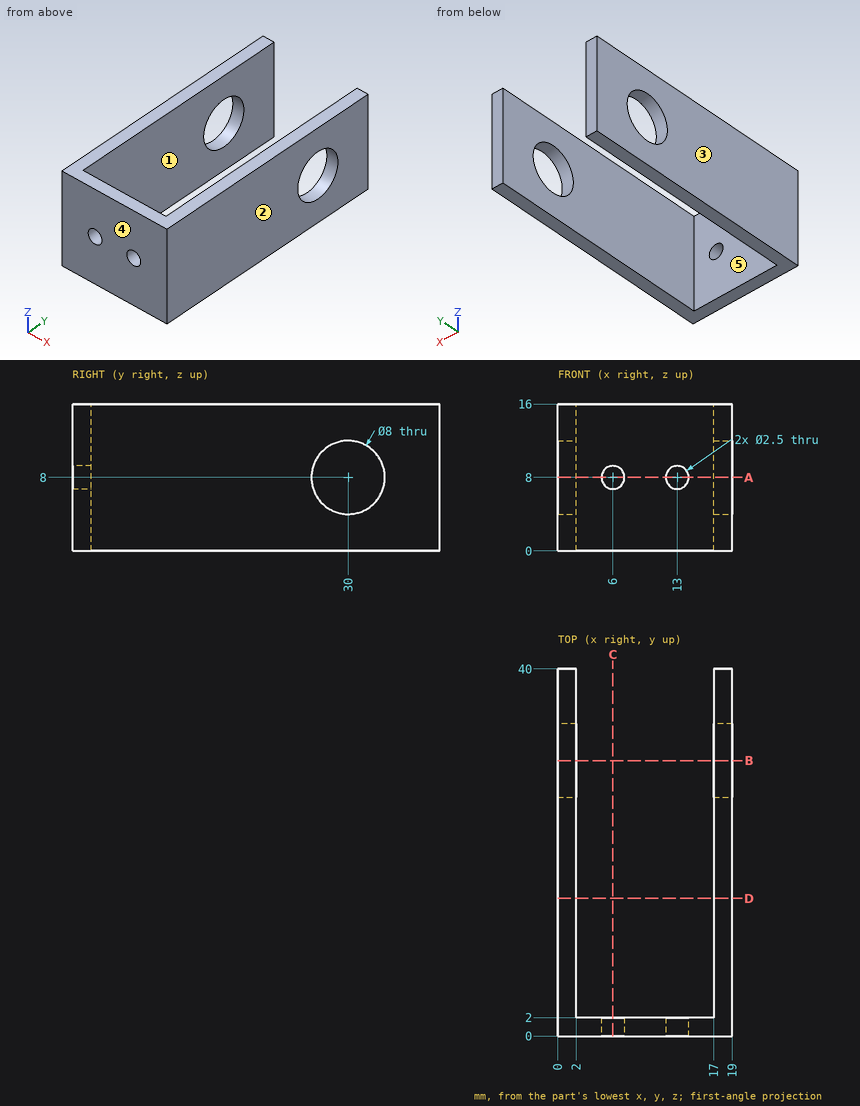
The figure shows three views and two pictorial views of one solid part (mm, origin at its lowest corner). Answer the questions. A direction names the side the tool comes from. Give positions to 0.01 mm unless a question says otherwise; leave off trailing zeros. Order: outer loops, then holes, each group sorted by start corner. A loop starts at its lowest first (then second) coordinate and runs counter-clockwise, first axis right, second up. Notation, with made-up numbers: M -26,81 L 7,81 A28 cw 7,115 Z; hole C 61.25,32.5 d8. An arc over 180 degrees is marked long. Return JSON: item names as keys, results as strings.
1) Section D-D, the plane y = 15 is taken. Write down the section's boundary in (x, z), plus the area to 3 significant figures.
Resolved:
{"outline": "M 0,0 L 2,0 L 2,16 L 0,16 Z; M 17,0 L 19,0 L 19,16 L 17,16 Z", "area": "64.0 mm^2"}
2) Section C-C, the plane x = 6 is taken. Write down the section's boundary in (y, z).
Resolved:
{"outline": "M 0,0 L 2,0 L 2,6.75 L 0,6.75 Z; M 0,9.25 L 2,9.25 L 2,16 L 0,16 Z"}
3) For a pull along X with two mould halves and no side action, classify the marked faces 3, 4 and 5 as +X half, -X half, draft (parallel to the pull), parting line (faces both ways), or undercut.
Resolved:
{"face 3": "-X half", "face 4": "draft", "face 5": "undercut"}
4) Section A-A, the plane z = 8 is taken. Write down the section's boundary in (x, y), plus the area to 3 significant figures.
Resolved:
{"outline": "M 0,0 L 4.75,0 L 4.75,2 L 2,2 L 2,26 L 0,26 Z; M 0,34 L 2,34 L 2,40 L 0,40 Z; M 7.25,0 L 11.75,0 L 11.75,2 L 7.25,2 Z; M 14.25,0 L 19,0 L 19,26 L 17,26 L 17,2 L 14.25,2 Z; M 17,34 L 19,34 L 19,40 L 17,40 Z", "area": "148 mm^2"}
5) Straight lines are drawn through the part: line 1 along Z through (x, y) = (17.65, 30); line 2 along X through (y, z) = (8, 8.25); line 3 along Y through (x, z) = (7, 10.5). For each, find the intervals that lie inside material, in ascending order. Write a range as [from, to].
Resolved:
{"line 1": "[0, 4], [12, 16]", "line 2": "[0, 2], [17, 19]", "line 3": "[0, 2]"}
6) A tool of negligible diameter and unlimited length cuts with its end or side. For the marked faces 1 and 2, from which of +Z, -Z, +X, -X, +Y, -Y can it reach the whole face along a straight path? Write none if from no direction.
Resolved:
{"face 1": "+Z, -Z, +Y", "face 2": "+Z, -Z, +X, +Y, -Y"}
7) Each of these flat-tipped pins is pushed along its axis until it touches: pin 1 (4 mm diameter, centred on x = 13, z = 7, fed in from +Y); pin 2 (4 mm diameter, centred on y = 29, z = 8, fed in from -X). Where does it stop, or does it pass through?
Resolved:
{"pin 1": "y = 2", "pin 2": "through"}
8) Section B-B, the plane y = 30 is taken. Write down the section's boundary in (x, z), plus the area to 3 significant figures.
Resolved:
{"outline": "M 0,0 L 2,0 L 2,4 L 0,4 Z; M 0,12 L 2,12 L 2,16 L 0,16 Z; M 17,0 L 19,0 L 19,4 L 17,4 Z; M 17,12 L 19,12 L 19,16 L 17,16 Z", "area": "32.0 mm^2"}
